```python
from build123d import *

# Parameters (mm, degrees)
SKETCH1_W           = 508
SKETCH1_H           = 101.6
BOSS_EXTRUDE1_DEPTH = 6.35
SKETCH2_R           = 25.4
SKETCH2_R_2         = 1.651
MOTOR_MOUNT_DEPTH   = 6.35
SKETCH3_R           = 9.525
CUT_EXTRUDE2_DEPTH  = 511.573170564
SKETCH4_R           = 3.175
CUT_EXTRUDE3_DEPTH  = 511.573170564
CUT_EXTRUDE4_DEPTH  = 511.573170564


with BuildPart() as part:
    # Sketch1 → Boss-Extrude1 (new body)
    with BuildSketch(Plane.XY):
        with Locations((254, 0)):
            Rectangle(SKETCH1_W, SKETCH1_H)
    extrude(amount=-BOSS_EXTRUDE1_DEPTH)

    # Sketch2 → Motor mount (cut)
    with BuildSketch(Plane.XY):
        with Locations((40.64, 0)):
            Circle(SKETCH2_R)
        with Locations((72.39, 0)):
            Circle(SKETCH2_R_2)
        with Locations((40.64, -31.75)):
            Circle(SKETCH2_R_2)
        with Locations((8.89, 0)):
            Circle(SKETCH2_R_2)
        with Locations((40.64, 31.75)):
            Circle(SKETCH2_R_2)
    extrude(amount=-MOTOR_MOUNT_DEPTH, mode=Mode.SUBTRACT)

    # Sketch3 → Cut-Extrude2 (cut, through all)
    with BuildSketch(Plane.XY):
        with Locations((112.0775, 0)):
            Circle(SKETCH3_R)
        with Locations((183.515, 0)):
            Circle(SKETCH3_R)
    extrude(amount=-CUT_EXTRUDE2_DEPTH, mode=Mode.SUBTRACT)

    # Sketch4 → Cut-Extrude3 (cut, through all)
    with BuildSketch(Plane.XY):
        with Locations((9.525, 41.275)):
            Circle(SKETCH4_R)
        with Locations((9.525, -41.275)):
            Circle(SKETCH4_R)
        with Locations((498.475, 41.275)):
            Circle(SKETCH4_R)
        with Locations((498.475, -41.275)):
            Circle(SKETCH4_R)
    extrude(amount=-CUT_EXTRUDE3_DEPTH, mode=Mode.SUBTRACT)

    # Sketch7 → Cut-Extrude4 (cut, through all)
    with BuildSketch(Plane.XY):
        with BuildLine():
            Line((85.406292789, 5.08), (92.341412089, 5.08))
            ThreePointArc((92.341412089, 5.08), (96.950572969, 6.134064693), (100.643442411, 9.08671294))
            ThreePointArc((100.643442411, 9.08671294), (112.0775, 14.605), (123.511557589, 9.08671294))
            ThreePointArc((123.511557589, 9.08671294), (127.204427031, 6.134064693), (131.813587911, 5.08))
            Line((131.813587911, 5.08), (162.585112959, 5.08))
            ThreePointArc((162.585112959, 5.08), (167.45975122, 6.214203951), (171.333000793, 9.383818205))
            ThreePointArc((171.333000793, 9.383818205), (184.777760897, 15.325227036), (197.068677539, 7.263261936))
            ThreePointArc((197.068677539, 7.263261936), (202.783248212, 4.735656121), (206.626270766, 9.662753319))
            Line((206.626270766, 9.662753319), (206.626270766, 31.603209647))
            ThreePointArc((206.626270766, 31.603209647), (203.520318205, 39.101642443), (196.02188541, 42.207595003))
            Line((196.02188541, 42.207595003), (25.263102588, 42.207595003))
            ThreePointArc((25.263102588, 42.207595003), (20.881723867, 41.260150637), (17.283250038, 38.587115578))
            add(Edge.make_bspline(
                [(17.283250038, 38.587115578), (11.530533455, 32.014027317), (16.787146308, 28.551640426), (21.263438452, 31.320883809)],
                knots=[0, 0, 0, 0, 1, 1, 1, 1], degree=3))
            ThreePointArc((21.263438452, 31.320883809), (52.918543043, 34.722993545), (75.39838363, 12.177999321))
            ThreePointArc((75.39838363, 12.177999321), (79.271558889, 7.034643814), (85.406292789, 5.08))
        make_face()
    cut_extrude4 = extrude(amount=-CUT_EXTRUDE4_DEPTH, mode=Mode.SUBTRACT)

    # Mirror1: Cut-Extrude4 across plane
    add(cut_extrude4.mirror(Plane.ZX), mode=Mode.SUBTRACT)


solid = part.part
```
The listing builds one solid part. Answer for the finished solid, in the listing's coordinates (mm). A direction names the side the tool comes from. Coordinates: 2 decimals unless noted, no trailing zeros.
Q1. Find the intervals of material crossed by line 1 along Y through (x, z) = (157.5, -0.5); line 2 along Y through (x, z) = (184.5, -2.5); line 3 along X through (y, z) = (15.5, -2.25), in increasing order.
Returned:
line 1: y = -50.8 to -42.21, -5.08 to 5.08, 42.21 to 50.8
line 2: y = -50.8 to -42.21, -15.35 to -9.47, 9.47 to 15.35, 42.21 to 50.8
line 3: x = 0 to 20.52, 60.76 to 74.05, 206.63 to 508
Q2. Which of the six approach directions +Z, -Z, +X, -X, +Y, -Y give full straight-line access (tool end or side, diameter ignored) to faces 3 (the flat face through (307, 1, -6.35)), 4 (the cylindrical face through (203.6, 39.02, -3.13))?
Returned:
face 3: -Z, +X, -X, +Y, -Y
face 4: +Z, -Z
Q3. The mould has two halves that part along X. Classify faces 1 (the flat face through (307, 1, 0)), 2 (the cylindrical face through (184.56, 15.34, -3.13)): released by +X, released by -X, zero draft, split by the parting line, or undercut.
Returned:
face 1: zero draft
face 2: undercut
Q4. Section A-A, the plane z = -3 is taken. Give the number of separate pieces and of enclosed holes in the cut face, then the cut area to 3 significant figures.
Returned:
separate pieces: 1
enclosed holes: 13
area: 38,800 mm2
